CAD build for the part. Positions are in the model's coordinates, mm. A direction names the side the tool comes from. Round coordinates to 2 decimals unless told otherwise and drop trailing zeros. Write each loop counter-clockwise with the first axis right and the second up, starting at its lowest first coordinate (ties: lowest second). Pieces come first, ordered by that corner, then holes. Notation, with made-up numbers: (-13, 83.25) -> (6, 83.25) arc R27 ccw to (6, 105.25) -> close; hole circle Ø8 at (9.25, 48). An arc over 180 degrees is marked (long way). Put each result on its own line as item: value. Start each with the question number.
1. Drill centre lines: line 1 (Z direction, x = -1, y = -5); line 2 (Z direction, x = -13.5, y = 2); line 3 (X direction, y = 0.25, z = 4). Where is each one in solid material? Low to high. Write a range as from..to.
2. 3-axis set-ups, long thin cutter, end or side, ignore diameter. For faces 1 (the cylindrical face through (-7.634, 0.088, 27.972)), 2 (the flat face through (5, 0, 19)), 3 (the flat face through (-14, 0, 17)), 4 (the flat face through (10.864, 0, 7)), 5 (the flat face through (-11.136, 0, 8)): which of +Z, -Z, +X, -X, +Y, -Y reach the whole face in a straight line?
3. Flat gauge pins, fed straight in: P1, Ø5.5, axis at y = 0.5, z = 24, coming from the +X side; P2, Ø2, axis at y = -4, z = 6, coming from the -X side; P3, Ø4, axis at y = 2.5, z = 6, coming from the +X side. Where does each tip first touch, or does it go through?
4. Saw through at B-B on z = 25.5. List the corners of the cut face in (x, y).
5. Saw through at D-D on y = 0. List the corners of the cut face in (x, z), and give its area (3 significant figures).
6. Saw through at A-A on y = 4.75. List the corners of the cut face in (x, z).
7. Saw through at C-C on x = 13. List the corners of the cut face in (y, z).
from build123d import *

# Parameters (mm, degrees)
F0_W     = 11.1358017506
F0_H     = 15
F0_W_2   = 10.8641982494
F0_H_2   = 2
F0_W_3   = 4.8641982494
F0_W_4   = 5.1358017506
F0_H_3   = 7
F1_DEPTH = 6.25
F2_R     = 2
F3_DEPTH = 11


with BuildPart() as f1:
    # F0 (on Front) → F1 (new body, symmetric)
    with BuildSketch(Plane.XZ):
        with Locations((-5.5679008753, 7.5)):
            Rectangle(F0_W, F0_H)
        with Locations((5.4320991247, 16)):
            Rectangle(F0_W_2, F0_H_2)
        with Locations((-5.5679008753, 16)):
            Rectangle(F0_W, F0_H_2)
        with Locations((-13.5679008753, 16)):
            Rectangle(F0_W_3, F0_H_2)
        with Locations((5.4320991247, 7.5)):
            Rectangle(F0_W_2, F0_H)
        with Locations((13.4320991247, 16)):
            Rectangle(F0_W_4, F0_H_2)
        with Locations((5.4320991247, 18)):
            Rectangle(F0_W_2, F0_H_2)
        with Locations((-5.5679008753, 22.5)):
            Rectangle(F0_W, F0_H_3)
        with Locations((-5.5679008753, 18)):
            Rectangle(F0_W, F0_H_2)
    extrude(amount=F1_DEPTH, both=True)

    # F2 (on face) → F3 (join)
    with BuildSketch(Plane.XY.offset(19)):
        with Locations((-5.6358017506, 0)):
            Circle(F2_R)
    extrude(amount=F3_DEPTH)


solid = f1.part
Return value:
1. line 1: z = 0..26
1. line 2: z = 15..17
1. line 3: x = -11.14..10.86
2. face 1: +Z
2. face 2: +Z, +X, +Y, -Y
2. face 3: +Z, -X, +Y, -Y
2. face 4: -Z, +X, +Y, -Y
2. face 5: -Z, -X, +Y, -Y
3. P1: stops at x = 0
3. P2: stops at x = -11.14
3. P3: stops at x = 10.86
4. outline: (-11.14, -6.25) -> (0, -6.25) -> (0, 6.25) -> (-11.14, 6.25) -> close
5. outline: (-16, 15) -> (-11.14, 15) -> (-11.14, 0) -> (10.86, 0) -> (10.86, 15) -> (16, 15) -> (16, 17) -> (10.86, 17) -> (10.86, 19) -> (0, 19) -> (0, 26) -> (-3.64, 26) -> (-3.64, 30) -> (-7.64, 30) -> (-7.64, 26) -> (-11.14, 26) -> (-11.14, 17) -> (-16, 17) -> close
5. area: 532 mm^2
6. outline: (-16, 15) -> (-11.14, 15) -> (-11.14, 0) -> (10.86, 0) -> (10.86, 15) -> (16, 15) -> (16, 17) -> (10.86, 17) -> (10.86, 19) -> (0, 19) -> (0, 26) -> (-11.14, 26) -> (-11.14, 17) -> (-16, 17) -> close
7. outline: (-6.25, 15) -> (6.25, 15) -> (6.25, 17) -> (-6.25, 17) -> close
